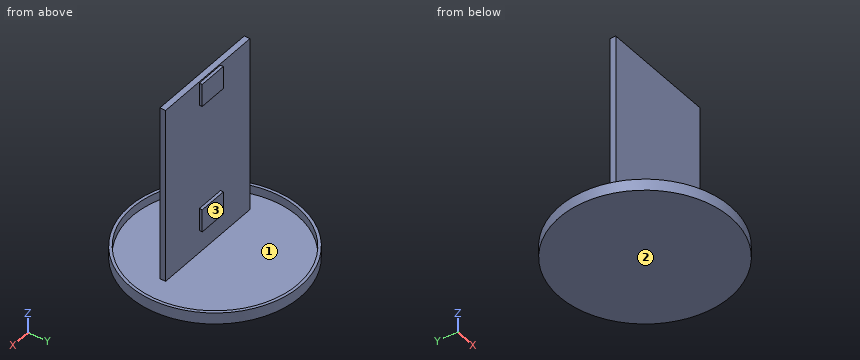
```python
from build123d import *

# Parameters (mm, degrees)
F0_R     = 75
F0_R_2   = 72.5
F1_DEPTH = 10
F2_DEPTH = 2.5
F3_W     = 100
F3_H     = 5
F4_DEPTH = 155
F5_W     = 25
F5_H     = 20
F6_DEPTH = 2.5
F7_W     = 25
F7_H     = 20
F8_DEPTH = 2.5


with BuildPart() as f1:
    # F0 (on Top) → F1 (new body)
    with BuildSketch(Plane.XY):
        Circle(F0_R)
        Circle(F0_R_2, mode=Mode.SUBTRACT)
    extrude(amount=F1_DEPTH)

    # F0 (on Top) → F2 (join)
    with BuildSketch(Plane.XY):
        Circle(F0_R_2)
    extrude(amount=F2_DEPTH)

    # F3 (on face) → F4 (join)
    with BuildSketch(Plane.XY.offset(2.5)):
        with Locations((-5, -12.5)):
            Rectangle(F3_W, F3_H)
    extrude(amount=F4_DEPTH)

    # F5 (on face) → F6 (join)
    with BuildSketch(Plane(origin=(0, -10, 0), x_dir=(-1, 0, 0), z_dir=(0, 1, 0))):
        with Locations((7.5, 32.5)):
            Rectangle(F5_W, F5_H)
    extrude(amount=F6_DEPTH)

    # F7 (on face) → F8 (join)
    with BuildSketch(Plane(origin=(0, -10, 0), x_dir=(-1, 0, 0), z_dir=(0, 1, 0))):
        with Locations((7.5, 146.25)):
            Rectangle(F7_W, F7_H)
    extrude(amount=F8_DEPTH)


solid = f1.part
```
Verification items for the finished model (mm, model axes). Face numbers are marked on the shaded views. Coordinates: 2 decimals unless noted, no trailing zeros. Write each loop counter-clockwise with the first axis right and the second up, starting at its lowest first coordinate (ties: lowest second). Pieces come first, ordered by that corner, then holes. Notation, with made-up numbers: (42.5, -34.75) - (98.5, -34.75) arc R19 ccw to (98.5, -11.75) - close; hole circle Ø5 at (-36.75, 72). An arc over 180 degrees is marked (long way). Write item = value, one per line.
Q1. Mould release check, pull along Y, two halves, no side actions. Record for the marked faces 1, 2 and 3: released by +Y, released by -Y, zero draft, split by the parting line, or undercut.
Answer:
face_1 = undercut
face_2 = zero draft
face_3 = released by +Y
Q2. Cross-section at D-D (x = -28). Enter the section's corners in (y, z), plus the area to 3 significant figures.
Answer:
outline = (-69.58, 0) - (69.58, 0) - (69.58, 10) - (66.87, 10) - (66.87, 2.5) - (-10, 2.5) - (-10, 157.5) - (-15, 157.5) - (-15, 2.5) - (-66.87, 2.5) - (-66.87, 10) - (-69.58, 10) - close
area = 1,160 mm²
Q3. Material ranges on L1, parallel to Y at x = 0, z = 4; L2, parallel to Y at x = -16, z = 46; L3, parallel to Z at x = 43.5, y = 12.5, recorded low to high. Write a range as from..to.
Answer:
L1 = -75..-72.5, -15..-10, 72.5..75
L2 = -15..-10
L3 = 0..2.5
Q4. Go/stop test with flat-tipped pins: pin 1 Ø0.8 at (y, z) = (-9, 143.5) entering from -X; pin 2 Ø5 at (x, y) = (-52.5, 5) entering from -Z; pin 3 Ø4 at (y, z) = (-12.5, 49) entering from -X; pin 4 Ø6 at (x, z) = (33.5, 110) entering from +Y. Record where each tip stops, or that it passes through.
Answer:
pin_1 = -20
pin_2 = 0
pin_3 = -55
pin_4 = -10
Q5. Cross-section at A-A (x = 0). Enter the section's corners in (y, z).
Answer:
outline = (-75, 0) - (75, 0) - (75, 10) - (72.5, 10) - (72.5, 2.5) - (-10, 2.5) - (-10, 22.5) - (-7.5, 22.5) - (-7.5, 42.5) - (-10, 42.5) - (-10, 136.25) - (-7.5, 136.25) - (-7.5, 156.25) - (-10, 156.25) - (-10, 157.5) - (-15, 157.5) - (-15, 2.5) - (-72.5, 2.5) - (-72.5, 10) - (-75, 10) - close
Q6. Cross-section at C-C (y = 54). Enter the section's corners in (x, z).
Answer:
outline = (-52.05, 0) - (52.05, 0) - (52.05, 10) - (48.38, 10) - (48.38, 2.5) - (-48.38, 2.5) - (-48.38, 10) - (-52.05, 10) - close
Q7. Cross-section at B-B (z = 38). Enter the section's corners in (x, y), plus the area to 4 significant figures.
Answer:
outline = (-55, -15) - (45, -15) - (45, -10) - (5, -10) - (5, -7.5) - (-20, -7.5) - (-20, -10) - (-55, -10) - close
area = 562.5 mm²
